Source: CAD feature listing. Evaluate the final solid. Frame: model axes, mm. A direction names the side the tool comes from. Round coordinates to 2 decimals unless told otherwise and drop trailing zeros. Write each loop counter-clockwise with the first axis right and the second up, starting at its lowest first coordinate (ties: lowest second). Pieces come first, ordered by that corner, then holes. Notation, with made-up numbers: M 3.5,11.5 L 61.5,11.5 A26 cw 61.5,40.5 Z; hole C 17.25,37 d11. An arc over 180 degrees is marked long. Answer in a Markdown table with one row per item. Add a question column.
Item 1: Material intervals for probe 1 along Z at (x, y) = (15, -5); probe 2 along Z at (x, y) = (0, -6.75); probe 3 along X at (y, z) = (-1.5, -6.95), sorted ascending.
Item 2: Cut plane B-B on y = -2.5. Return loops of the section in (x, z), and give its area (3 significant figures).
Item 3: Cut plane C-C on z = 0. Return loops of the section in (x, y) (3 decimals), and give its area (3 significant figures).
Item 4: Set-up query: faces 5 (the face through (14, -6, 0)), 6 (the face through (0, 41, -1)), 7 (the face through (0, 45.237, 0)). Return all of +Z, -Z, +X, -X, +Y, -Y with unobstructed straight access to the full face (end or side cutting, diameter ignored); none if empty.
Item 5: Cut plane D-D on y = 14. Return loops of the section in (x, z), and give its area (3 significant figures).
Item 6: Contact query for flat-ended pins moving along their axis: pin 1 (1.5 mm diameter, centred on x = 13.5, z = -6.5, fed in from -Y); pin 2 (4.5 mm diameter, centred on x = -1, y = -26.5, fed in from +Z); pin 3 (3.5 mm diameter, centred on x = 0.5, z = 15, fed in from -Y); pin 4 (6 mm diameter, centred on x = 2.5, z = -10, fed in from -Y). Output: stop coordinate, or through.
Item 7: Mould query, pull axis Z, two halves, no side actions, for faces 1 (the face through (-0.65, -22.61, -9.88)), 2 (the face through (-8.08, -6.2, -11.96)), 3 (the face through (15, -3.246, 0)), 4 (the face through (0, -9.246, 0)). Classes: released by +Z, released by -Z, zero draft, split by the parting line, or undercut.
from build123d import *

# Parameters (mm, degrees)
SCHIZZO1_W                   = 18.5
SCHIZZO1_H                   = 18.4912
SCHIZZO2_R                   = 6
ESTRUSIONE_ESTRUSIONE1_DEPTH = 4.572
SCHIZZO3_R                   = 3
ESTRUSIONE_ESTRUSIONE2_DEPTH = 17.83
TAGLIO_ESTRUSIONE1_DEPTH     = 11.98
SCHIZZO5_R                   = 16.5
ESTRUSIONE_ESTRUSIONE3_DEPTH = 23.2918
SCHIZZO6_R                   = 4.445
ESTRUSIONE_ESTRUSIONE4_DEPTH = 4
SCHIZZO7_R                   = 1
ESTRUSIONE_ESTRUSIONE5_DEPTH = 8.7
FORO_3_0_3_1_D               = 3
FORO_3_0_3_1_DEPTH           = 6
FORO_3_0_3_2_D               = 3
FORO_3_0_3_2_DEPTH           = 10


with BuildPart() as part:
    # Schizzo1 → Rivoluzione1 (revolve)
    with BuildSketch(Plane(origin=(0, 0, 0), x_dir=(-1, 0, 0), z_dir=(0, 0, -1))):
        with Locations((-9.25, 0)):
            Rectangle(SCHIZZO1_W, SCHIZZO1_H)
    revolve(axis=Axis((0, -9.2456, 0), (0, 1, 0)))

    # Schizzo2 → Estrusione-Estrusione1 (add)
    with BuildSketch(Plane.XZ.offset(9.2456)):
        with Locations((0, -6.95)):
            Circle(SCHIZZO2_R)
    extrude(amount=ESTRUSIONE_ESTRUSIONE1_DEPTH)

    # Schizzo3 → Estrusione-Estrusione2 (add)
    with BuildSketch(Plane.XZ.offset(13.8176)):
        with Locations((0, -6.95)):
            Circle(SCHIZZO3_R)
    extrude(amount=ESTRUSIONE_ESTRUSIONE2_DEPTH)

    # Schizzo4 → Taglio-Estrusione1 (cut)
    with BuildSketch(Plane.XZ.offset(31.6476)):
        with BuildLine():
            Line((-2.821661699, -5.931066609), (2.821661699, -5.931066609))
            ThreePointArc((2.821661699, -5.931066609), (0, -3.95), (-2.821661699, -5.931066609))
        make_face()
    extrude(amount=-TAGLIO_ESTRUSIONE1_DEPTH, mode=Mode.SUBTRACT)

    # Schizzo5 → Estrusione-Estrusione3 (add)
    with BuildSketch(Plane(origin=(0, 9.2456, 0), x_dir=(-1, 0, 0), z_dir=(0, 1, 0))):
        Circle(SCHIZZO5_R)
    extrude(amount=ESTRUSIONE_ESTRUSIONE3_DEPTH)

    # Schizzo6 → Estrusione-Estrusione4 (add)
    with BuildSketch(Plane(origin=(0, 32.5374, 0), x_dir=(-1, 0, 0), z_dir=(0, 1, 0))):
        Circle(SCHIZZO6_R)
    extrude(amount=ESTRUSIONE_ESTRUSIONE4_DEPTH)

    # Schizzo7 → Estrusione-Estrusione5 (add)
    with BuildSketch(Plane(origin=(0, 36.5374, 0), x_dir=(-1, 0, 0), z_dir=(0, 1, 0))):
        Circle(SCHIZZO7_R)
    extrude(amount=ESTRUSIONE_ESTRUSIONE5_DEPTH)

    # Foro Ø3.0 (3)-1
    with Locations(Plane(origin=(0, -9.2456, 0), x_dir=(-1, 0, 0), z_dir=(0, -1, 0))):
        with Locations((15.5, 0), (7.75, -13.423393759), (-15.5, 0), (7.75, 13.423393759)):
            Hole(FORO_3_0_3_1_D / 2, depth=FORO_3_0_3_1_DEPTH)

    # Foro Ø3.0 (3)-2
    with Locations(Plane(origin=(0, -9.2456, 0), x_dir=(-1, 0, 0), z_dir=(0, -1, 0))):
        with Locations((13.8545119, 6.95), (-13.8545119, 6.95), (0, -15.5)):
            Hole(FORO_3_0_3_2_D / 2, depth=FORO_3_0_3_2_DEPTH)


solid = part.part
Results below:
| question | item | result |
|---|---|---|
| 1 | probe 1 | -10.83 to -7.92, -5.98 to -1.41, 1.41 to 10.83 |
| 1 | probe 2 | -18.5 to 14, 17 to 18.5 |
| 1 | probe 3 | -17.14 to -15.35, -12.35 to 12.35, 15.35 to 17.14 |
| 2 | outline | C 0,0 d37; hole C -13.85,-6.95 d3; hole C 0,15.5 d3; hole C 13.85,-6.95 d3 |
| 2 | area | 1,050 mm2 |
| 3 | outline | M -18.5,-9.246 L -17,-9.246 L -17,-3.246 L -14,-3.246 L -14,-9.246 L 14,-9.246 L 14,-3.246 L 17,-3.246 L 17,-9.246 L 18.5,-9.246 L 18.5,9.246 L 16.5,9.246 L 16.5,32.537 L 4.445,32.537 L 4.445,36.537 L 1,36.537 L 1,45.237 L -1,45.237 L -1,36.537 L -4.445,36.537 L -4.445,32.537 L -16.5,32.537 L -16.5,9.246 L -18.5,9.246 Z |
| 3 | area | 1,470 mm2 |
| 4 | face 5 | -Y |
| 4 | face 6 | +Y |
| 4 | face 7 | +Z, -Z, +X, -X, +Y |
| 5 | outline | C 0,0 d33 |
| 5 | area | 855 mm2 |
| 6 | pin 1 | y = 0.75 |
| 6 | pin 2 | z = -5.93 |
| 6 | pin 3 | y = -9.25 |
| 6 | pin 4 | y = -31.65 |
| 7 | face 1 | split by the parting line |
| 7 | face 2 | undercut |
| 7 | face 3 | undercut |
| 7 | face 4 | zero draft |
